Can you work these out from the model? Positions are in its coordinate system, mm. A direction names the side the tool comes from. Give positions to 0.01 mm unless a question says otherwise; leave off trailing zeros. Order: outer loops, then holes, each group sorted by start corner. A loop starts at its lowest first (then second) coordinate and runs counter-clockwise, first axis right, second up. Notation, with made-up numbers: M 49.5,54 L 97.5,54 A30 cw 97.5,90 Z; hole C 34.5,-2.75 d8. An arc over 180 degrees is marked long. One line per question, with ' | ' between items. Start each with the question number.
1) If we section it at C-C, the plane x = 24: Please give me the cut outline in (y, z), plus the area to 3 significant figures.
2) If we section it at A-A, the plane y = 25: Please give me the cut outline in (x, z).
3) Please list where these lines run through material, in increasing order: line 1 along Y through (x, z) = (5.5, 0); line 2 along Y through (x, z) = (17, 2); line 3 along X through (y, z) = (4, -5.5). Write a range as [from, to].
4) If we section it at D-D, the plane z = 0: Please give me the cut outline in (x, y).
5) For faces 1 (the cylindrical face through (1.785, 37.699, -5.967)), 2 (the cylindrical face through (31.8, 6.1, 4.5)), 3 (the flat face through (24, 8, 2)), 4 (the cylindrical face through (6.215, 37.699, -5.967)), which set-ups out of +Z, -Z, +X, -X, +Y, -Y let a thin tool reach every point of the face, with its end or its side?
6) I'm going to push flat-ended pins straight in: pin 1 Ø1.5 at (x, z) = (4, -6) entering from -Y; pin 2 Ø1.4 at (y, z) = (20, -5) entering from -X; pin 3 Ø4 at (x, z) = (23, 5.5) entering from +Y. Where does each tip first touch, or does it pass through?
7) If we section it at B-B, the plane y = 3: Please give me the cut outline in (x, z).
```python
from build123d import *

# Parameters (mm, degrees)
BOSS_EXTRUDE1_DEPTH = 4
BOSS_EXTRUDE2_DEPTH = 29
CHAMFER1_SIZE       = 4
CHAMFER2_SIZE       = 6
CUT_EXTRUDE1_REACH  = 40
SKETCH3_R           = 2.5
CUT_EXTRUDE2_REACH  = 34
SKETCH4_R           = 2.5
SKETCH5_W           = 5
SKETCH5_H           = 5.8
BOSS_EXTRUDE3_DEPTH = 27
FILLET1_R           = 2
FILLET2_R           = 1


with BuildPart() as part:
    # Sketch1 → Boss-Extrude1 (new body, symmetric)
    with BuildSketch(Plane.XY):
        Polygon((0, 0), (0, 38), (8, 38), (8, 8), (32, 8), (32, 0), align=None)
    extrude(amount=BOSS_EXTRUDE1_DEPTH, both=True)

    # Sketch2 → Boss-Extrude2 (add)
    with BuildSketch(Plane(origin=(32, 0, 0), x_dir=(0, 0, -1), z_dir=(1, 0, 0))):
        Polygon((-4, 6.5), (-9.8, 6.5), (-9.8, 1.5), (-4, 0), align=None)
        Polygon((4, 0), (4, 6.5), (9.8, 6.5), (9.8, 1.5), align=None)
    extrude(amount=-BOSS_EXTRUDE2_DEPTH)

    # Chamfer1
    chamfer1_edges = [part.edges().sort_by_distance(p)[0] for p in [
        (3, 4, 9.8),
        (32, 4, 9.8),
        (3, 4, -9.8),
        (32, 4, -9.8),
    ]]
    chamfer(chamfer1_edges, length=CHAMFER1_SIZE)

    # Chamfer2
    chamfer2_edges = [part.edges().sort_by_distance(p)[0] for p in [
        (8, 8, 0),
    ]]
    chamfer(chamfer2_edges, length=CHAMFER2_SIZE)

    # Sketch3 → Cut-Extrude1 (cut, up to next)
    with BuildSketch(Plane.XZ, mode=Mode.PRIVATE) as cut_extrude1_sk1:
        with Locations((22, 0)):
            Circle(SKETCH3_R)
    cut_extrude1_tool1 = extrude(cut_extrude1_sk1.sketch, amount=-CUT_EXTRUDE1_REACH, mode=Mode.PRIVATE) & part.part
    add(cut_extrude1_tool1.solids().sort_by_distance((22, 0, 0))[0], mode=Mode.SUBTRACT)

    # Sketch4 → Cut-Extrude2 (cut, up to next)
    with BuildSketch(Plane.ZY, mode=Mode.PRIVATE) as cut_extrude2_sk1:
        with Locations((0, 25)):
            Circle(SKETCH4_R)
    cut_extrude2_tool1 = extrude(cut_extrude2_sk1.sketch, amount=-CUT_EXTRUDE2_REACH, mode=Mode.PRIVATE) & part.part
    add(cut_extrude2_tool1.solids().sort_by_distance((0, 25, 0))[0], mode=Mode.SUBTRACT)

    # Sketch5 → Boss-Extrude3 (add)
    with BuildSketch(Plane(origin=(0, 38, 0), x_dir=(1, 0, 0), z_dir=(0, 1, 0))):
        with Locations((4, 6.9)):
            Rectangle(SKETCH5_W, SKETCH5_H)
        with Locations((4, -6.9)):
            Rectangle(SKETCH5_W, SKETCH5_H)
    extrude(amount=-BOSS_EXTRUDE3_DEPTH)

    # Fillet1
    fillet1_edges = [part.edges().sort_by_distance(p)[0] for p in [
        (4, 38, 9.8),
        (4, 11, -9.8),
        (4, 38, -9.8),
        (4, 11, 9.8),
    ]]
    fillet(fillet1_edges, radius=FILLET1_R)

    # Fillet2
    fillet2_edges = [part.edges().sort_by_distance(p)[0] for p in [
        (1.5, 38, 5.9),
        (6.5, 24.5, -9.8),
        (0, 0, 0),
        (1.5, 24.5, -9.8),
        (0, 38, 0),
        (1.5, 38, -5.9),
        (8, 38, 0),
        (1.5, 11, -5.9),
        (1.5, 37.414213562, -9.214213562),
        (1.5, 11.585786438, -9.214213562),
        (32, 8, 0),
        (6.5, 37.414213562, -9.214213562),
        (6.5, 11.585786438, -9.214213562),
        (32, 0, 0),
        (1.5, 24.5, 9.8),
        (6.5, 24.5, 9.8),
        (6.5, 38, 5.9),
        (6.5, 11, 5.9),
        (6.5, 37.414213562, 9.214213562),
        (6.5, 11.585786438, 9.214213562),
        (1.5, 37.414213562, 9.214213562),
        (1.5, 11.585786438, 9.214213562),
        (32, 7.25, 4),
        (7.25, 38, 4),
        (32, 6.5, 4.9),
        (32, 7.25, -4),
        (32, 0.232758621, -4.9),
        (17.5, 1.5, -9.8),
        (17.5, 6.5, -9.8),
        (28, 4, -9.8),
        (7, 4, -9.8),
        (32, 6.5, -4.9),
        (30, 6.5, -7.8),
        (5, 6.5, -7.8),
        (3, 3.482758621, -5.8),
        (30, 0.982758621, -7.8),
        (5, 0.982758621, -7.8),
        (17.5, 6.5, 9.8),
        (17.5, 1.5, 9.8),
        (28, 4, 9.8),
        (7, 4, 9.8),
        (32, 0.232758621, 4.9),
        (30, 0.982758621, 7.8),
        (5, 0.982758621, 7.8),
        (3, 3.482758621, 5.8),
        (30, 6.5, 7.8),
        (5, 6.5, 7.8),
        (32, 3.482758621, 5.8),
        (32, 3.482758621, -5.8),
        (7.25, 38, -4),
        (0.75, 38, -4),
        (6.5, 11, -5.9),
        (6.5, 38, -5.9),
        (0.75, 38, 4),
        (1.5, 11, 5.9),
    ]]
    fillet(fillet2_edges, radius=FILLET2_R)


solid = part.part
```
Results found:
1) outline: M 0,-4 L 1.31,-9.05 A1 ccw 2.27,-9.8 L 5.5,-9.8 A1 ccw 6.5,-8.8 L 6.5,-4 L 8,-4 L 8,-1.5 L 0,-1.5 Z; M 0,1.5 L 8,1.5 L 8,4 L 6.5,4 L 6.5,8.8 A1 ccw 5.5,9.8 L 2.27,9.8 A1 ccw 1.31,9.05 L 0,4 Z | area: 106 mm²
2) outline: M 0,-4 L 1.5,-4 L 1.5,-8.8 A1 ccw 2.5,-9.8 L 5.5,-9.8 A1 ccw 6.5,-8.8 L 6.5,-4 L 8,-4 L 8,-2.5 L 0,-2.5 Z; M 0,2.5 L 8,2.5 L 8,4 L 6.5,4 L 6.5,8.8 A1 ccw 5.5,9.8 L 2.5,9.8 A1 ccw 1.5,8.8 L 1.5,4 L 0,4 Z
3) line 1: y = [0, 22.5], [27.5, 38] | line 2: y = [0, 8] | line 3: x = [3.01, 31.99]
4) outline: M 0,1 A1 ccw 1,0 L 19.5,0 L 19.5,8 L 14,8 L 8,14 L 8,22.5 L 0,22.5 Z; M 0,27.5 L 8,27.5 L 8,37 A1 ccw 7,38 L 1,38 A1 ccw 0,37 Z; M 24.5,0 L 31,0 A1 ccw 32,1 L 32,7 A1 ccw 31,8 L 24.5,8 Z
5) face 1: -Z, -X, +Y | face 2: +Z, +X, +Y | face 3: +Z, -Z, +X, +Y | face 4: -Z, +X, +Y
6) pin 1: stops at y = 0.32 | pin 2: stops at x = 1.5 | pin 3: stops at y = 8
7) outline: M 0,-4 L 3,-4 L 3,-5.39 A1 ccw 3.29,-6.09 L 6.71,-9.51 A1 ccw 7.41,-9.8 L 27.59,-9.8 A1 ccw 28.29,-9.51 L 31.71,-6.09 A1 ccw 32,-5.39 L 32,5.39 A1 ccw 31.71,6.09 L 28.29,9.51 A1 ccw 27.59,9.8 L 7.41,9.8 A1 ccw 6.71,9.51 L 3.29,6.09 A1 ccw 3,5.39 L 3,4 L 0,4 Z; hole C 22,0 d5
